Input: part model. Units: mm. Frame: model coordinates. Coordinates: 2 decimals unless noted, no trailing zeros. Order: outer loops, then holes, each group sorted by start corner. A loop starts at its lowest first (then second) coordinate and runs counter-clockwise, first axis right, second up. Notation, with made-up numbers: M 68.25,64 L 115.25,64 A10 cw 115.25,78 Z; hole C 89.5,-16.75 d2. An arc over 180 degrees is marked long. One line per item, written item: value.
```python
from build123d import *

# Parameters (mm, degrees)
SKETCH_1_R               = 13.5
SKETCH_1_R_2             = 3.25
SKETCH_1_R_3             = 1.6
EXTRUDE_3_DEPTH          = 2
EXTRUDE_4_DEPTH          = 2
PATTERN_CIRCULAR_1_COUNT = 6
CUT_EXTRUDE_1_REACH      = 60
SKETCH_2_R               = 1.6
PATTERN_CIRCULAR_2_COUNT = 6


with BuildPart() as part:
    # Sketch 1 → Extrude 3 (new body)
    with BuildSketch(Plane.XY):
        Circle(SKETCH_1_R)
        Circle(SKETCH_1_R_2, mode=Mode.SUBTRACT)
        with Locations((6.5, 0)):
            Circle(SKETCH_1_R_3, mode=Mode.SUBTRACT)
        with Locations((-6.5, 0)):
            Circle(SKETCH_1_R_3, mode=Mode.SUBTRACT)
    extrude(amount=EXTRUDE_3_DEPTH)

    # Sketch 1_7 → Extrude 4 (add)
    with BuildSketch(Plane.XY):
        with BuildLine():
            Line((37.187130839, 21.47), (11.691342951, 6.75))
            ThreePointArc((11.691342951, 6.75), (12.473550673, 5.163383929), (13.041589791, 3.488113492))
            Line((13.041589791, 3.488113492), (38.937130839, 18.438911087))
            Line((38.937130839, 18.438911087), (37.187130839, 21.47))
        make_face()
        with BuildLine():
            ThreePointArc((9.541589791, 9.550291318), (10.708396989, 8.220719794), (11.691342951, 6.75))
            Line((11.691342951, 6.75), (37.187130839, 21.47))
            Line((37.187130839, 21.47), (35.437130839, 24.501088913))
            Line((35.437130839, 24.501088913), (9.541589791, 9.550291318))
        make_face()
    extrude_4 = extrude(amount=EXTRUDE_4_DEPTH)

    # Pattern Circular 1: Extrude 4 ×6 about axis
    pattern_circular_1_axis = Axis((0, 0, 0), (0, 0, 1))
    for i in range(1, PATTERN_CIRCULAR_1_COUNT):
        add(extrude_4.rotate(pattern_circular_1_axis, i * 360 / PATTERN_CIRCULAR_1_COUNT))

    # Sketch 2 → Cut-Extrude 1 (cut, up to next)
    with BuildSketch(Plane.XY.offset(2), mode=Mode.PRIVATE) as cut_extrude_1_sk1:
        with Locations((32.85700382, 18.97)):
            Circle(SKETCH_2_R)
    cut_extrude_1_tool1 = extrude(cut_extrude_1_sk1.sketch, amount=-CUT_EXTRUDE_1_REACH, mode=Mode.PRIVATE) & part.part
    cut_extrude_1 = cut_extrude_1_tool1.solids().sort_by_distance((32.857004, 18.97, 2))[0]
    add(cut_extrude_1, mode=Mode.SUBTRACT)

    # Pattern Circular 2: Cut-Extrude 1 ×6 about axis
    pattern_circular_2_axis = Axis((0, 0, 0), (0, 0, 1))
    for i in range(1, PATTERN_CIRCULAR_2_COUNT):
        add(cut_extrude_1.rotate(pattern_circular_2_axis, i * 360 / PATTERN_CIRCULAR_2_COUNT), mode=Mode.SUBTRACT)


solid = part.part
```
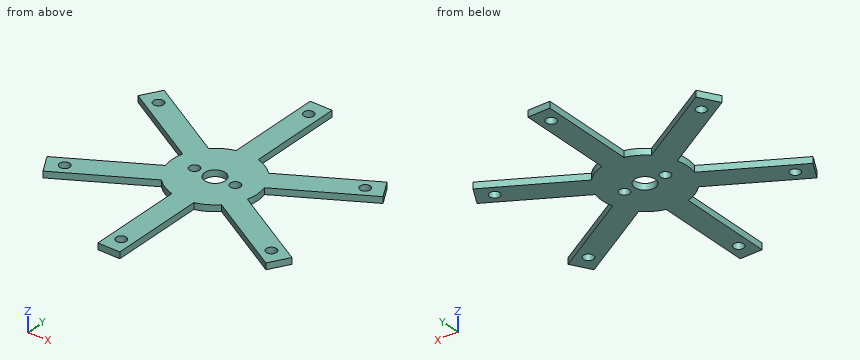
(1) Ray query, line 1 (Y direction, x = 0, z = 1.45); line 2 (X direction, y = -18.97, z = 0.95); line 3 (Y direction, x = -0.5, z = 1.6). Return the intervals inside material, ascending. Write a range as from..to.
Data:
line 1: y = -42.94..-39.54, -36.34..-3.25, 3.25..36.34, 39.54..42.94
line 2: x = -38.63..-34.46, -31.26..-25.86, -3.5..3.5, 25.86..31.26, 34.46..38.63
line 3: y = -42.94..-39.46, -36.42..-3.21, 3.21..36.42, 39.46..42.94
(2) Cut plane C-C on y = 0. Output: boundary loops of the cut face in (x, z).
Data:
outline: M -13.5,0 L -8.1,0 L -8.1,2 L -13.5,2 Z; M -4.9,0 L -3.25,0 L -3.25,2 L -4.9,2 Z; M 3.25,0 L 4.9,0 L 4.9,2 L 3.25,2 Z; M 8.1,0 L 13.5,0 L 13.5,2 L 8.1,2 Z
(3) Cut plane A-A on y = -37.94. Output: boundary loops of the cut face in (x, z), plus the area to 3 significant figures.
Data:
outline: M -3.5,0 L -1.6,0 L -1.6,2 L -3.5,2 Z; M 1.6,0 L 3.5,0 L 3.5,2 L 1.6,2 Z
area: 7.60 mm2
(4) Cut plane B-B on x = 22. Output: boundary loops of the cut face in (y, z), plus the area to 3 significant figures.
Data:
outline: M -16.74,0 L -8.66,0 L -8.66,2 L -16.74,2 Z; M 8.66,0 L 16.74,0 L 16.74,2 L 8.66,2 Z
area: 32.3 mm2
(5) Cut plane D-D on z = 1.55. Give the number of separate pieces and of enclosed holes in the cut face, plus the area to 3 significant figures.
Data:
separate pieces: 1
enclosed holes: 9
area: 1,720 mm2
(6) First-contact query: pin 1 (3 mm diameter, centred on x = 5.5, y = 23.5, fed in from -Z); pin 2 (5 mm diameter, centred on x = 15.5, y = 2.5, fed in from -Z); pin 3 (1 mm diameter, centred on y = 28.5, z = 1.5, fed in from +X); pin 4 (1 mm diameter, centred on y = -23.5, z = 1, fed in from -X). Flat tips, straight axial feed; report the tip coordinate or a pass-through.
Data:
pin 1: passes through
pin 2: stops at z = 0
pin 3: stops at x = 3.5
pin 4: stops at x = -36.3
